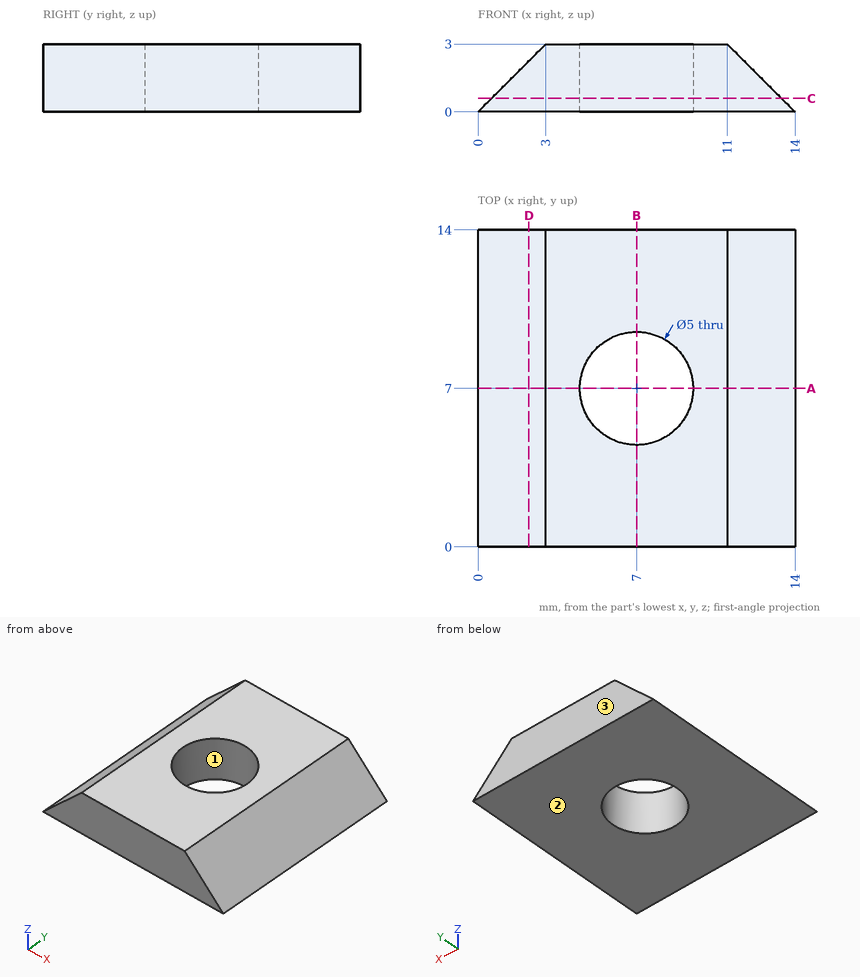
Study the drawing (mm; zero at the part's minimum x, y, z) and answer. Coordinates: 2 decimals unless noted, no trailing zeros. Write each loop counter-clockwise with the first axis right and the second up, starting at its lowest first coordinate (ties: lowest second). Pieces come first, ordered by that corner, then holes. Notation, with made-up numbers: (-6.5, -29) - (42.5, -29) arc R24 cw to (42.5, -1) - close; hole circle Ø1 at (8.5, 64.5). An arc over 180 degrees is marked (long way). One line per question, with ' | ' between items.
1) Find section A-A, the plane y = 7. Determine the outline of the cut face in (x, z), and give its area (3 significant figures).
Checks:
outline: (0, 0) - (4.5, 0) - (4.5, 3) - (3, 3) - close; (9.5, 0) - (14, 0) - (11, 3) - (9.5, 3) - close | area: 18.0 mm2
2) Find section D-D, the plane x = 2.25. Determine the outline of the cut face in (y, z), and give its area (3 significant figures).
Checks:
outline: (0, 0) - (14, 0) - (14, 2.25) - (0, 2.25) - close | area: 31.5 mm2
3) The mould has two halves that part along Y. Classify the marked faces 1, 2 and 3: +Y half, -Y half, draft (parallel to the pull), parting line (faces both ways), or undercut.
Checks:
face 1: undercut | face 2: draft | face 3: +Y half
4) Find section B-B, the plane x = 7. Determine the outline of the cut face in (y, z).
Checks:
outline: (0, 0) - (4.5, 0) - (4.5, 3) - (0, 3) - close; (9.5, 0) - (14, 0) - (14, 3) - (9.5, 3) - close
5) Consider probe 1 along Y at (x, z) = (7, 2.15); probe 2 along Y at (x, z) = (8, 2.2); probe 3 along X at (y, z) = (6.75, 1.05). Determine where each line is inside the solid, lowest interval first. Write a range as [from, to].
Checks:
probe 1: [0, 4.5], [9.5, 14] | probe 2: [0, 4.71], [9.29, 14] | probe 3: [1.05, 4.51], [9.49, 12.95]
6) Find section C-C, the plane z = 0.6. Determine the outline of the cut face in (x, y), and give its area (3 significant figures).
Checks:
outline: (0.6, 0) - (13.4, 0) - (13.4, 14) - (0.6, 14) - close; hole circle Ø5 at (7, 7) | area: 160 mm2
7) A flat-ended cylindrical pin translates along its axis: P1, Ø1.5, axis at y = 11, z = 2.5, coming from the +X side. Find the tip coordinate at first contact, or state that the pin passes through.
Checks:
P1: x = 12.25
